Autodesk Inventor part; units mm, degrees
ref_plane "YZ Plane" through (0, 0, 0) normal (1, 0, 0) x (0, 1, 0)
ref_plane "XZ Plane" through (0, 0, 0) normal (0, 1, 0) x (-1, 0, 0)
ref_plane "XY Plane" through (0, 0, 0) normal (0, 0, 1) x (1, 0, 0)
sketch "Sketch1" plane through (0, 0, 0) normal (0, 0, 1) x (1, 0, 0)
  line L0 (-20, 3.175) -> (20, 3.175)
  line L1 (20, 3.175) -> (20, -3.175)
  line L2 (20, -3.175) -> (-20, -3.175)
  line L3 (-20, -3.175) -> (-20, 3.175)
  line L4 (0, 10.7485) -> (0, -11.1125)
  point P0 (0, 0)
  dimension "d5" = 40
extrude "Extrusion1" add sketch "Sketch1" along normal blind 40
sketch "Sketch2" plane through (0, 0, 0) normal (0, 1, 0) x (-1, 0, 0)
  circle A0 centre (0, 20) radius 7.9375
  circle A1 centre (0, 20) radius 9.525
  line L0 (20, 0) -> (-20, 0)
  point P0 (0, 0)
  dimension "d2" = 15.875
  dimension "d6" = 20
extrude "Extrusion2" add sketch "Sketch2" against normal blind 10
properties part number "BindingPiece1"
Model file for the job. Use its own axes, mm. A direction names the side the tool comes from. Give positions to 0.01 mm unless a question says otherwise; leave off trailing zeros. Loops run counter-clockwise (first coordinate to the right, second up) from the corner with the lowest first, then second, coordinate; pieces in that order, holes last.
Item 1: Drop flat-ended pins along their axis: P1, Ø2, axis at y = -7, z = 11.5, coming from the -X side; P2, Ø8, axis at x = 8.5, z = 5.5, coming from the -Y side (3 decimals). Give the stop position or say it passes through.
Check values:
P1: stops at x = -5.87
P2: stops at y = -3.175
Item 2: Drill centre lines: line 1 along Z through (x, y) = (0, -8) (1 decimal); line 2 along Y through (x, z) = (-8, 34) (3 decimals); line 3 along X through (y, z) = (-4, 22). Where is each one in solid material? Low to high.
Check values:
line 1: z = 10.5 to 12.1, 27.9 to 29.5
line 2: y = -3.175 to 3.175
line 3: x = -9.31 to -7.68, 7.68 to 9.31
Item 3: Which spindle directions (+Z, -Z, +X, -X, +Y, -Y) get a long thin tool onto all of the face, cutting with end or side? Do faces 4 (the face through (0, -3.175, 20)), 5 (the face through (20, 0, 20)). Say none if no direction does.
Check values:
face 4: -Y
face 5: +Z, -Z, +X, +Y, -Y
Item 4: Slice it at C-C (z = 20). Write the cut outline in (x, y) (1 decimal).
Check values:
outline: (-20, -3.2) - (-9.5, -3.2) - (-9.5, -10) - (-7.9, -10) - (-7.9, -3.2) - (7.9, -3.2) - (7.9, -10) - (9.5, -10) - (9.5, -3.2) - (20, -3.2) - (20, 3.2) - (-20, 3.2) - close
Item 5: Slice it at D-D (z = 4.5). Write the cut outline in (x, y) (3 decimals), plus the area to 3 significant figures.
Check values:
outline: (-20, -3.175) - (20, -3.175) - (20, 3.175) - (-20, 3.175) - close
area: 254 mm2
Item 6: Slice it at A-A (x = 0). Write the cut outline in (y, z) (1 decimal), plus the area to 3 significant figures.
Check values:
outline: (-10, 10.5) - (-3.2, 10.5) - (-3.2, 0) - (3.2, 0) - (3.2, 40) - (-3.2, 40) - (-3.2, 29.5) - (-10, 29.5) - (-10, 27.9) - (-3.2, 27.9) - (-3.2, 12.1) - (-10, 12.1) - close
area: 276 mm2
Item 7: Mould opens along X. For faces 1 (the face through (0, 0, 0)), 2 (the face through (1.03, -6.54, 27.87)), 3 (the face through (2.06, -6.54, 10.7)) say: +X half, -X half, draft (parallel to the pull), parting line (faces both ways), or undercut.
Check values:
face 1: draft
face 2: undercut
face 3: parting line
